Can you work these out from the drawing? Everything is in mm from the part's minimum corner. A direction names the side the tool comes from. Coordinates: 2 decimals unless noted, no trailing zeros. Loops run counter-clockwise (first coordinate to the right, second up) from the corner with the lowest first, then second, coordinate; pieces in that order, holes last. Notation, with made-up numbers: (38.25, 68.5) -> (58.25, 68.5) arc R25 ccw to (58.25, 103.5) -> close; hole circle Ø2 at (39.5, 11). An arc over 180 degrees is marked (long way). One line per question, with ' | ' between items.
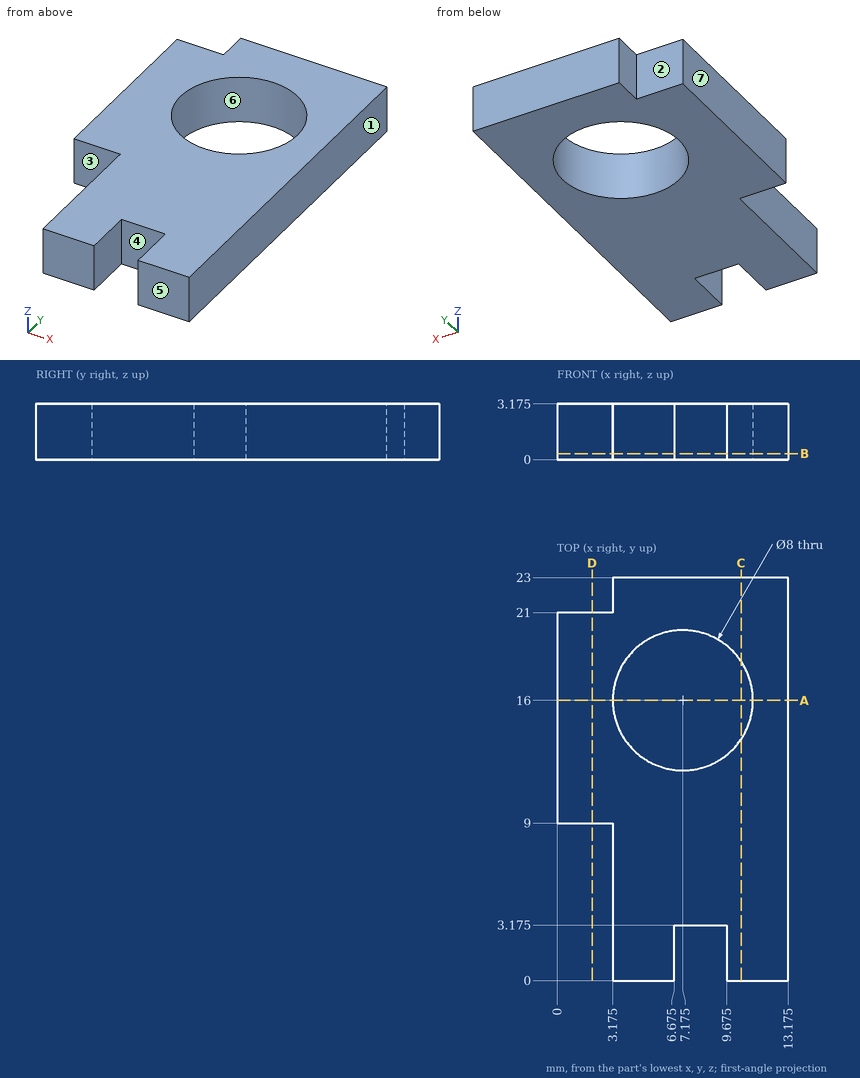
Q1. Imagine slicing it at D-D on x = 2. Write out the boundary of the cut face in (y, z) (3 decimals).
Values follow:
outline: (9, 0) -> (21, 0) -> (21, 3.175) -> (9, 3.175) -> close
Q2. For pin 1 (1 mm diameter, centred on y = 1.5, z = 1.5, fed in from -X) (3 decimals); pin 2 (1 mm diameter, centred on x = 1.5, z = 1.5, fed in from -Y), each with a flat end and sliding along its axis, tell me the tip position at first contact or that it passes through.
Values follow:
pin 1: stops at x = 3.175 | pin 2: stops at y = 9
Q3. Imagine slicing it at A-A on y = 16. Write out the boundary of the cut face in (x, z) (3 decimals), plus the area to 3 significant figures.
Values follow:
outline: (0, 0) -> (3.175, 0) -> (3.175, 3.175) -> (0, 3.175) -> close; (11.175, 0) -> (13.175, 0) -> (13.175, 3.175) -> (11.175, 3.175) -> close | area: 16.4 mm2
Q4. For the marked faces 1, 2, 3 and 4, which set-ups out of +Z, -Z, +X, -X, +Y, -Y let a thin tool reach every point of the face, with its end or its side?
Values follow:
face 1: +Z, -Z, +X, +Y, -Y | face 2: +Z, -Z, -X, +Y | face 3: +Z, -Z, -X, -Y | face 4: +Z, -Z, -Y
Q5. Imagine slicing it at C-C on x = 10.5. Write out the boundary of the cut face in (y, z) (3 decimals).
Values follow:
outline: (0, 0) -> (13.776, 0) -> (13.776, 3.175) -> (0, 3.175) -> close; (18.224, 0) -> (23, 0) -> (23, 3.175) -> (18.224, 3.175) -> close
Q6. We'd pull the mould along Y, two halves only. Please class the marked faces 5, 6 and 7: released by +Y, released by -Y, zero draft, split by the parting line, or undercut.
Values follow:
face 5: released by -Y | face 6: undercut | face 7: zero draft
Q7. Imagine slicing it at B-B on z = 0.35. Write out the boundary of the cut face in (x, y) (3 decimals).
Values follow:
outline: (0, 9) -> (3.175, 9) -> (3.175, 0) -> (6.675, 0) -> (6.675, 3.175) -> (9.675, 3.175) -> (9.675, 0) -> (13.175, 0) -> (13.175, 23) -> (3.175, 23) -> (3.175, 21) -> (0, 21) -> close; hole circle Ø8 at (7.175, 16)
Q8. Please list where these lines run through material, in increasing order: L1, parallel to X at y = 2, z = 1.6 (3 decimals); L2, parallel to X at y = 3.5, z = 2.65 (3 decimals); L3, parallel to Y at x = 1.25, z = 1. Write a range as [from, to].
Values follow:
L1: x = [3.175, 6.675], [9.675, 13.175] | L2: x = [3.175, 13.175] | L3: y = [9, 21]
